```python
from build123d import *

# Parameters (mm, degrees)
F1_DEPTH = 16
F2_R     = 2.5
F3_DEPTH = 10
F4_R     = 3.5
F5_DEPTH = 11
F6_R     = 1.99999
F7_W     = 9.5
F7_H     = 3.5
F8_DEPTH = 12.3
F9_R     = 5


# Not quite as in the source:
# - a fillet or chamfer is up to 0.001 mm smaller than in the source, because OpenCascade refuses the exact size


with BuildPart() as f1:
    # F0 (on Top) → F1 (new body)
    with BuildSketch(Plane.XY):
        Polygon((-5.5, -2.8019716907), (-5.5, -26), (-2, -26), (-2, -7.4497503303), (2, -7.4497503303), (2, -26), (5.5, -26), (5.5, -2.8019716907), (8, -2.8019716907), (8, 9.1980283093), (5.5, 10.9290892892), (-5.5, 10.9290892892), (-8, 9.1980283093), (-8, -2.8019716907), align=None)
    extrude(amount=F1_DEPTH)

    # F2 (on face) → F3 (cut)
    with BuildSketch(Plane(origin=(0, 10.9290892892, 0), x_dir=(-1, 0, 0), z_dir=(0, 1, 0))):
        with Locations((0, 9)):
            Circle(F2_R)
    extrude(amount=-F3_DEPTH, mode=Mode.SUBTRACT)

    # F4 (on face) → F5 (cut, through all)
    with BuildSketch(Plane.YZ.offset(5.5)):
        with Locations((-18, 8)):
            Circle(F4_R)
    extrude(amount=-F5_DEPTH, mode=Mode.SUBTRACT)

    # F6 (radius 2 in the source; OpenCascade refuses exactly that, so slightly less here)
    f6_edges = [f1.edges().sort_by_distance(p)[0] for p in [
        (-5.5, -2.801972, 8),
        (2, -7.44975, 8),
        (-2, -7.44975, 8),
        (5.5, -2.801972, 8),
    ]]
    fillet(f6_edges, radius=F6_R)

    # F7 (on face) → F8 (cut)
    with BuildSketch(Plane.XY.offset(16)):
        with Locations((0, 6.1790892892)):
            Rectangle(F7_W, F7_H)
    extrude(amount=-F8_DEPTH, mode=Mode.SUBTRACT)

    # F9
    f9_edges = [f1.edges().sort_by_distance(p)[0] for p in [
        (3.75, -26, 16),
        (3.75, -26, 0),
        (-3.75, -26, 16),
        (-3.75, -26, 0),
    ]]
    fillet(f9_edges, radius=F9_R)


solid = f1.part
```
The model under review builds one solid part; all positions refer to its coordinate system, in mm. A direction names the side the tool comes from. Give positions to 0.01 mm unless a question says otherwise; leave off trailing zeros. Write each loop counter-clockwise with the first axis right and the second up, starting at its lowest first coordinate (ties: lowest second). Pieces come first, ordered by that corner, then holes. Notation, with made-up numbers: M 48,-20 L 66,-20 A12 cw 66,-15 Z; hole C 51.5,76.25 d1. An arc over 180 degrees is marked long. Answer in a Markdown table with one row per item.
Item 1: Add section A-A on y = -12. Give the boundary of the cut face in (x, z).
Check sheet entries:
| item | result |
|---|---|
| outline | M -5.5,0 L -2,0 L -2,16 L -5.5,16 Z; M 2,0 L 5.5,0 L 5.5,16 L 2,16 Z |
Item 2: For P1, Ø0.6, axis at x = 7.5, z = 7.5, coming from the -Y side; P2, Ø8, axis at y = -17, z = 10, coming from the -X side; P3, Ø5, axis at y = -14.5, z = 6, coming from the +X side, all flat-tipped, find the tip position at first contact; note any pin that passes through.
Check sheet entries:
| item | result |
|---|---|
| P1 | y = -2.82 |
| P2 | x = -5.5 |
| P3 | x = 5.5 |
Item 3: For line 1 along X through (y, z) = (6, 14.5); line 2 along X through (y, z) = (-13.5, 3.75); line 3 along Z through (x, y) = (0, 9.85), list the stretches that pass through material, from the lowest coordinate up.
Check sheet entries:
| item | result |
|---|---|
| line 1 | -8 to -4.75, 4.75 to 8 |
| line 2 | -5.5 to -2, 2 to 5.5 |
| line 3 | 0 to 6.5, 11.5 to 16 |
Item 4: Add section D-D on x = -1.5. Give the boundary of the cut face in (y, z).
Check sheet entries:
| item | result |
|---|---|
| outline | M -8.13,0 L 10.93,0 L 10.93,7 L 7.93,7 L 7.93,3.7 L 4.43,3.7 L 4.43,7 L 0.93,7 L 0.93,11 L 4.43,11 L 4.43,16 L -8.13,16 Z; M 7.93,11 L 10.93,11 L 10.93,16 L 7.93,16 Z |
Item 5: Add section B-B on y = -18. Give the boundary of the cut face in (x, z).
Check sheet entries:
| item | result |
|---|---|
| outline | M -5.5,0 L -2,0 L -2,4.5 L -5.5,4.5 Z; M -5.5,11.5 L -2,11.5 L -2,16 L -5.5,16 Z; M 2,0 L 5.5,0 L 5.5,4.5 L 2,4.5 Z; M 2,11.5 L 5.5,11.5 L 5.5,16 L 2,16 Z |
Item 6: Tool access review of faces 1 (the face through (5.5, -13, 8)), 2 (the face through (0, 0.929, 9)), 3 (the face through (-5.5, -13, 8)): name each direction out of +Z, -Z, +X, -X, +Y, -Y from which nothing blocks a thin tool from reaching the whole face with its end or side.
Check sheet entries:
| item | result |
|---|---|
| face 1 | +Z, -Z, +X, -Y |
| face 2 | +Y |
| face 3 | +Z, -Z, -X, -Y |
Item 7: Draft analysis for pull direction Z (two halves, no side actions). For faces 4 (the face through (-4, -24, 1)), 5 (the face through (-8, 3, 8)), 6 (the face through (0.54, 9.45, 6.56)), state which applies: +Z half, -Z half, draft (parallel to the pull), parting line (faces both ways), or undercut.
Check sheet entries:
| item | result |
|---|---|
| face 4 | -Z half |
| face 5 | draft |
| face 6 | undercut |
